from build123d import *

# Parameters (mm, degrees)
F0_R     = 12.5
F1_DEPTH = 65
F2_R     = 5
F3_R     = 8
F4_DEPTH = 20
F5_SIZE  = 0.5
F6_R     = 3
F7_DEPTH = 20


with BuildPart() as f1:
    # F0 (on Top) → F1 (new body)
    with BuildSketch(Plane.XY):
        Circle(F0_R)
    extrude(amount=F1_DEPTH)

    # F2
    f2_edges = [f1.edges().sort_by_distance(p)[0] for p in [
        (-12.5, 0, 65),
    ]]
    fillet(f2_edges, radius=F2_R)

    # F3 (on face) → F4 (join)
    with BuildSketch(Plane(origin=(0, 0, 0), x_dir=(1, 0, 0), z_dir=(0, 0, -1))):
        Circle(F3_R)
    extrude(amount=F4_DEPTH)

    # F5
    f5_edges = [f1.edges().sort_by_distance(p)[0] for p in [
        (-8, 0, -20),
        (-8, 0, 0),
    ]]
    chamfer(f5_edges, length=F5_SIZE)

    # F6 (on Front) → F7 (cut, symmetric)
    with BuildSketch(Plane.XZ):
        with Locations((0, 55)):
            Circle(F6_R)
    extrude(amount=F7_DEPTH, both=True, mode=Mode.SUBTRACT)


solid = f1.part
Input: part model. Units: mm. Frame: model coordinates. A direction names the side the tool comes from. Give positions to 0.01 mm unless a question says otherwise; leave off trailing zeros. Loops run counter-clockwise (first coordinate to the right, second up) from the corner with the lowest first, then second, coordinate; pieces in that order, holes last. Notation, with made-up numbers: M 46.5,67 L 67.5,67 A26 ccw 67.5,92 Z; hole C -5.5,30 d7. An arc over 180 degrees is marked long. Use one line per item in the form item = value.
1. First-contact query: pin 1 (1 mm diameter, centred on x = 1, z = -6, fed in from -Y); pin 2 (5 mm diameter, centred on x = 7.5, z = -4.5, fed in from +Y) (3 decimals); pin 3 (2 mm diameter, centred on y = 9, z = 16.5, fed in from +X). Flat tips, straight axial feed; report the tip coordinate or a pass-through.
Numbers:
pin_1 = -7.98
pin_2 = 6.245
pin_3 = 9.6
2. Reachability of faces 4 (the face through (11.923, 3.755, 29.58)), 5 (the face through (-3, -8.2, 0)) from +Z, -Z, +X, -X, +Y, -Y: full face, straight path, thin tool, end or side. Return the list, or none.
Numbers:
face_4 = +Z, -Z
face_5 = -Z
3. Section query C-C, the plane z = 55. Return the cut outline in (x, y), and give its area (3 significant figures).
Numbers:
outline = M -3,-12.13 L -3,12.13 A12.5 ccw Z; M 3,-12.13 A12.5 ccw 3,12.13 Z
area = 342 mm²
4. Line query: L1, parallel to Z at x = 0, y = -5; L2, parallel to X at y = 0.5, z = 37; L3, parallel to Z at x = -1.25, y = 5.75. Output: solid intervals per line, ascending.
Numbers:
L1 = -20 to 52, 58 to 65
L2 = -12.49 to 12.49
L3 = -20 to 52.27, 57.73 to 65
5. Section query B-B, the plane y = 0. Return the cut outline in (x, z).
Numbers:
outline = M -12.5,0 L -8.5,0 L -8,-0.5 L -8,-19.5 L -7.5,-20 L 7.5,-20 L 8,-19.5 L 8,-0.5 L 8.5,0 L 12.5,0 L 12.5,60 A5 ccw 7.5,65 L -7.5,65 A5 ccw -12.5,60 Z; hole C 0,55 d6
6. Section query D-D, the plane z = -7. Return the cut outline in (x, y).
Numbers:
outline = C 0,0 d16
7. Pull-direction query (X, two-part tool) for faces 1 (the face through (0, 0, -20)), 2 (the face through (-1.73, 7.81, -9.87)), 3 (the face through (0, 0, 58)); classes: released by +X, released by -X, zero draft, split by the parting line, or undercut.
Numbers:
face_1 = zero draft
face_2 = split by the parting line
face_3 = undercut
8. Section query A-A, the plane x = 0. Return the cut outline in (y, z).
Numbers:
outline = M -12.5,0 L -8.5,0 L -8,-0.5 L -8,-19.5 L -7.5,-20 L 7.5,-20 L 8,-19.5 L 8,-0.5 L 8.5,0 L 12.5,0 L 12.5,52 L -12.5,52 Z; M -12.5,58 L 12.5,58 L 12.5,60 A5 ccw 7.5,65 L -7.5,65 A5 ccw -12.5,60 Z
